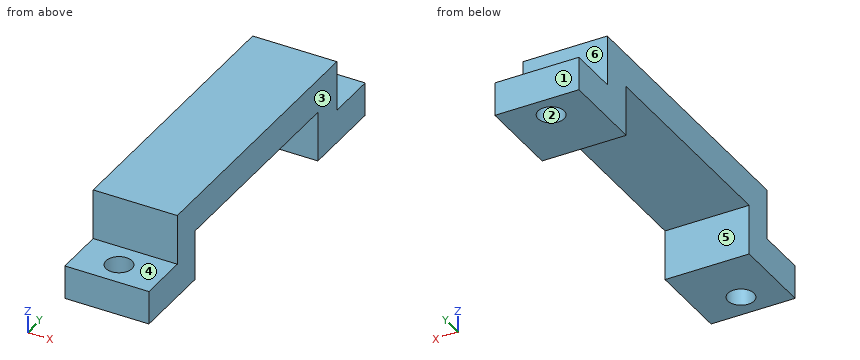
```python
from build123d import *

# Parameters (mm, degrees)
F0_W     = 6
F0_H     = 4
F0_W_2   = 26
F1_DEPTH = 10
F3_D     = 3.1


with BuildPart() as f1:
    # F0 (on Right) → F1 (new body)
    with BuildSketch(Plane.YZ):
        Polygon((-8.098859, -4), (-8.098859, 0), (-11.832699, 0), (-11.832699, -6), (-11.832699, -10), (-8.098859, -10), align=None)
        with Locations((-14.832699, -8)):
            Rectangle(F0_W, F0_H)
        with Locations((4.901141, -2)):
            Rectangle(F0_W_2, F0_H)
        Polygon((21.901141, 0), (17.901141, 0), (17.901141, -4), (17.901141, -10), (21.901141, -10), (21.901141, -6), align=None)
        with Locations((24.901141, -8)):
            Rectangle(F0_W, F0_H)
    extrude(amount=F1_DEPTH)

    # F3 (through all)
    with Locations(Plane.XY):
        with Locations((4.781065, -14.87558), (4.865282, 25.127819)):
            Hole(F3_D / 2)


solid = f1.part
```
Source: CAD feature listing. Evaluate the final solid. Frame: model axes, mm. Face numbers are marked on the shaded views. A direction names the side the tool comes from. Give positions to 0.01 mm unless a question says otherwise; leave off trailing zeros. Loops run counter-clockwise (first coordinate to the right, second up) from the corner with the lowest first, then second, coordinate; pieces in that order, holes last. Notation, with made-up numbers: (66, 83) - (75, 83) arc R29 cw to (75, 110) - close; hole circle Ø1 at (69.25, -33). An arc over 180 degrees is marked (long way). Use CSV: the item, a comma, the result in double quotes.
1) Cut plane C-C (x = 3.75). Output: boundary loops of the cut face in (y, z).
Worked out:
outline,"(-17.83, -10) - (-16.03, -10) - (-16.03, -6) - (-17.83, -6) - close; (-13.72, -10) - (-8.1, -10) - (-8.1, -4) - (17.9, -4) - (17.9, -10) - (24.05, -10) - (24.05, -6) - (21.9, -6) - (21.9, 0) - (-11.83, 0) - (-11.83, -6) - (-13.72, -6) - close; (26.2, -10) - (27.9, -10) - (27.9, -6) - (26.2, -6) - close"
2) Set-up query: the marked faces 4, 5 and 6. Return all of +Z, -Z, +X, -X, +Y, -Y with unobstructed straight access to the full face (end or side cutting, diameter ignored); none if empty.
Worked out:
face 4,"+Z, +X, -X, -Y"
face 5,"-Z, +X, -X"
face 6,"+Z, +X, -X, +Y"
3) Line query: line 1 (Y direction, x = 5.5, z = -7.5); line 2 (Y direction, x = 7, z = -5.75); line 3 (Y direction, x = 9.25, z = -9.25). Output: solid intervals per line, ascending.
Worked out:
line 1,"y = -17.83 to -16.25, -13.5 to -8.1, 17.9 to 23.71, 26.54 to 27.9"
line 2,"y = -11.83 to -8.1, 17.9 to 21.9"
line 3,"y = -17.83 to -8.1, 17.9 to 27.9"
4) Cut plane A-A (z = -5.5). Output: boundary loops of the cut face in (x, y), and give its area (3 significant figures).
Worked out:
outline,"(0, -11.83) - (10, -11.83) - (10, -8.1) - (0, -8.1) - close; (0, 17.9) - (10, 17.9) - (10, 21.9) - (0, 21.9) - close"
area,"77.3 mm^2"
5) Pin query (flat end, axial travel): P1, Ø5, axis at x = 4, z = -5.5, coming from the +Y side; P2, Ø5, axis at x = 4, y = -16, coming from the +Z side; P3, Ø3, axis at x = 6, z = -3.5, coming from the +Y side; P4, Ø5, axis at x = 5.5, y = 10, coming from the -Z side. Return the tip coordinate at first contact, or that it passes through.
Worked out:
P1,"stops at y = 27.9"
P2,"stops at z = -6"
P3,"stops at y = 21.9"
P4,"stops at z = -4"
6) Cut plane B-B (x = 9.25). Output: boundary loops of the cut face in (y, z), and give its area (3 significant figures).
Worked out:
outline,"(-17.83, -10) - (-8.1, -10) - (-8.1, -4) - (17.9, -4) - (17.9, -10) - (27.9, -10) - (27.9, -6) - (21.9, -6) - (21.9, 0) - (-11.83, 0) - (-11.83, -6) - (-17.83, -6) - close"
area,"229 mm^2"
7) Mould query, pull axis X, two halves, no side actions, for the marked faces 1, 2 and 3. Classes: +X half, -X half, draft (parallel to the pull), parting line (faces both ways), or undercut.
Worked out:
face 1,"draft"
face 2,"undercut"
face 3,"+X half"
8) Cut plane D-D (y = 11). Output: boundary loops of the cut face in (x, z).
Worked out:
outline,"(0, -4) - (10, -4) - (10, 0) - (0, 0) - close"
